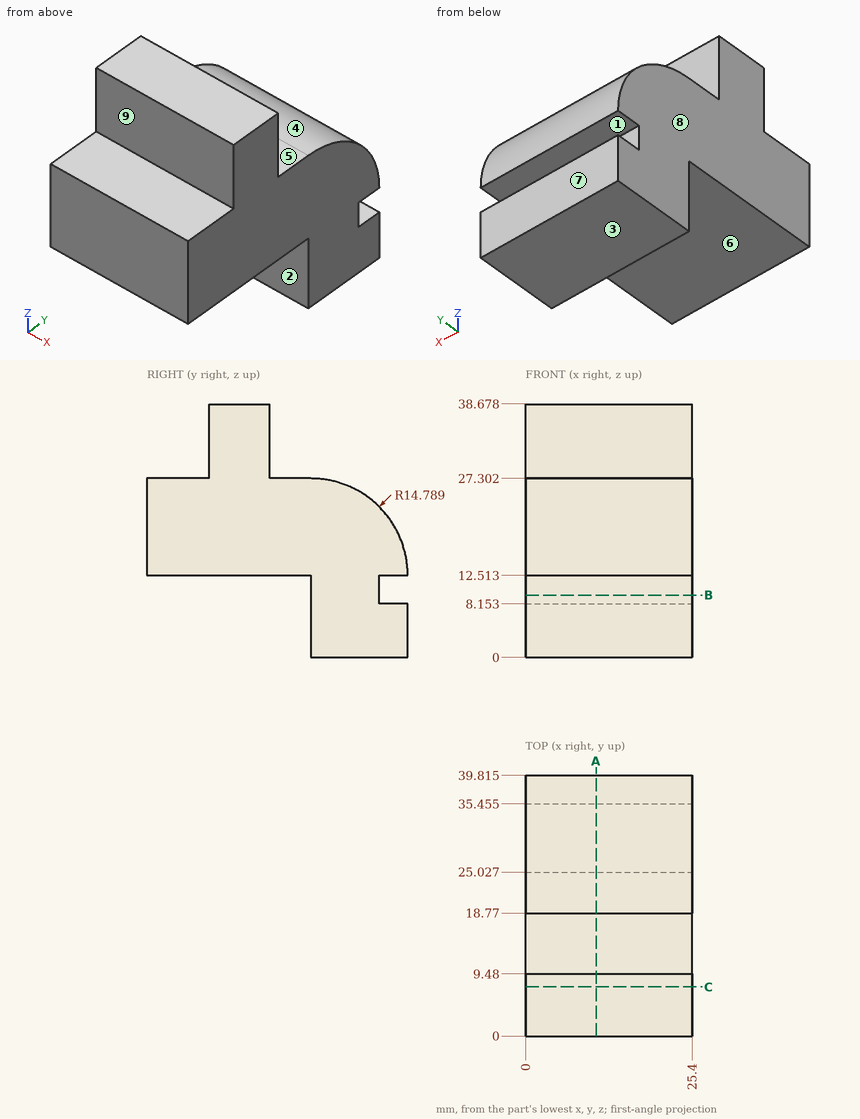
Design review of the part shown in the three views and the two pictorial views. Dimensions are in mm from the part's minimum x, y and z. A direction names the side the tool comes from. Coordinates: 2 decimals unless noted, no trailing zeros. Order: outer loops, then holes, each group sorted by start corner. A loop starts at its lowest first (then second) coordinate and runs counter-clockwise, first axis right, second up.
1) Clearance check with flat-ended pins moving along their axes: pin 1 (12.5 mm diameter, centred on x = 14.5, z = 34, fed in from +Y); pin 2 (5 mm diameter, centred on x = 10.5, y = 22.5, fed in from +Z); pin 3 (6.5 mm diameter, centred on x = 10.5, z = 6.5, fed in from -Y). State where each tip first meets the part, or that it passes through.
2) For the marked faces 5, 6, 7, 8 and 9, list the 3-axis set-ups (+Z, -Z, +X, -X, +Y, -Y) from which the entire face can be reached by the end or side of a thin tool; tool diameter is ignored.
3) Take a section at C-C, the plane y = 7.5. Give the boundary of the cut face in (x, z).
4) Mouldability with a two-part tool opening along Z and no side actions: class the marked faces 1, 2, 3 and 4 as +Z half, -Z half, draft (parallel to the pull), parting line (faces both ways), or undercut.
5) Wall thickness on line 1 along Z through (x, y) = (9.5, 5); line 2 along Y through (x, z) = (13.25, 7) (1 decimal); line 3 along Z through (x, y) = (22.5, 13.5): over which ranges is each line inside the solid? List them lowest first.
6) Take a section at A-A, the plane x = 10.75. Give the boundary of the cut face in (y, z) (1 decimal).
7) Take a section at B-B, the plane z = 9.5. Give the boundary of the cut face in (x, y) (1 decimal), and give its area (3 significant figures).
Returned:
1. pin 1: stops at y = 18.77
1. pin 2: stops at z = 27.3
1. pin 3: stops at y = 25.03
2. face 5: +Z, +X, -X, +Y
2. face 6: -Z, +X, -X, -Y
2. face 7: +Z, -Z, +X, -X, +Y
2. face 8: +Z, -Z, -X, +Y, -Y
2. face 9: +Z, +X, -X, -Y
3. outline: (0, 12.51) - (25.4, 12.51) - (25.4, 27.3) - (0, 27.3) - close
4. face 1: undercut
4. face 2: draft
4. face 3: -Z half
4. face 4: +Z half
5. line 1: z = 12.51 to 27.3
5. line 2: y = 25 to 39.8
5. line 3: z = 12.51 to 38.68
6. outline: (0, 12.5) - (25, 12.5) - (25, 0) - (39.8, 0) - (39.8, 8.2) - (35.5, 8.2) - (35.5, 12.5) - (39.8, 12.5) arc R14.8 ccw to (25, 27.3) - (18.8, 27.3) - (18.8, 38.7) - (9.5, 38.7) - (9.5, 27.3) - (0, 27.3) - close
7. outline: (0, 25) - (25.4, 25) - (25.4, 35.5) - (0, 35.5) - close
7. area: 265 mm2
